```python
from build123d import *

# Parameters (mm, degrees)
F0_R     = 11.049
F1_DEPTH = 6.35


with BuildPart() as f1:
    # F0 (on Top) → F1 (new body)
    with BuildSketch(Plane.XY):
        with BuildLine():
            ThreePointArc((30.5423546194, 13.9698608404), (19.000422111, 19.0038325132), (13.9698381707, 30.547241977))
            ThreePointArc((13.9698381707, 30.547241977), (13.9699595426, 30.5136210859), (13.97, 30.48))
            ThreePointArc((13.97, 30.48), (9.8782817373, 20.6017182709), (1.15e-08, 16.51))
            ThreePointArc((1.15e-08, 16.51), (11.6743329615, 11.6743329533), (16.51, 0))
            ThreePointArc((16.51, 0), (20.623788609, 9.900302875), (30.5423546194, 13.9698608404))
        make_face()
        with BuildLine():
            ThreePointArc((1.15e-08, 16.51), (-9.8782817291, 20.6017182627), (-13.97, 30.48))
            ThreePointArc((-13.97, 30.48), (-18.9768088864, 19.0202694582), (-30.4173910664, 13.969859703))
            ThreePointArc((-30.4173910664, 13.969859703), (-20.5796074118, 9.8561212756), (-16.51, 0))
            ThreePointArc((-16.51, 0), (-11.6743329533, 11.6743329615), (1.15e-08, 16.51))
        make_face()
        with BuildLine():
            ThreePointArc((-30.4173910664, 13.969859703), (-40.3361211962, 9.9003926673), (-44.45, 2.241e-07))
            ThreePointArc((-44.45, 2.241e-07), (-40.2581741683, -9.9773849246), (-30.1982875449, -13.9671592707))
            ThreePointArc((-30.1982875449, -13.9671592707), (-20.5026149969, -9.7781740883), (-16.51, 0))
            ThreePointArc((-16.51, 0), (-20.5796074118, 9.8561212756), (-30.4173910664, 13.969859703))
        make_face()
        with Locations((-30.48, 0)):
            Circle(F0_R, mode=Mode.SUBTRACT)
        with BuildLine():
            ThreePointArc((-30.1982875449, -13.9671592707), (-18.895154623, -19.0895439026), (-13.97, -30.48))
            ThreePointArc((-13.97, -30.48), (-9.8782817214, -20.6017182551), (3.33e-08, -16.51))
            ThreePointArc((3.33e-08, -16.51), (-11.6743329456, -11.6743329692), (-16.51, 0))
            ThreePointArc((-16.51, 0), (-20.5026149969, -9.7781740883), (-30.1982875449, -13.9671592707))
        make_face()
        with BuildLine():
            ThreePointArc((13.9686715274, -30.6726545055), (18.8427220321, -19.1504715121), (30.2294023882, -13.9677521755))
            ThreePointArc((30.2294023882, -13.9677521755), (20.5135124382, -9.7892811626), (16.51, 0))
            ThreePointArc((16.51, 0), (11.6743329692, -11.6743329456), (3.33e-08, -16.51))
            ThreePointArc((3.33e-08, -16.51), (9.8782817449, -20.6017182786), (13.97, -30.48))
            ThreePointArc((13.97, -30.48), (13.9696678779, -30.5763295429), (13.9686715274, -30.6726545055))
        make_face()
        with BuildLine():
            ThreePointArc((3.33e-08, -16.51), (11.6743329692, -11.6743329456), (16.51, 0))
            Line((16.51, 0), (11.049, 0))
            ThreePointArc((11.049, 0), (7.8128228253, -7.8128228253), (0, -11.049))
            Line((0, -11.049), (0, -16.51))
        make_face()
        with BuildLine():
            Line((11.049, 0), (16.51, 0))
            ThreePointArc((16.51, 0), (11.6743329615, 11.6743329533), (1.15e-08, 16.51))
            Line((0, 16.51), (0, 11.049))
            ThreePointArc((0, 11.049), (7.8128228253, 7.8128228253), (11.049, 0))
        make_face()
        with BuildLine():
            Line((0, 11.049), (0, 16.51))
            ThreePointArc((1.15e-08, 16.51), (-11.6743329533, 11.6743329615), (-16.51, 0))
            Line((-16.51, 0), (-11.049, 0))
            ThreePointArc((-11.049, 0), (-7.8128228253, 7.8128228253), (0, 11.049))
        make_face()
        with BuildLine():
            ThreePointArc((-16.51, 0), (-11.6743329456, -11.6743329692), (3.33e-08, -16.51))
            Line((0, -16.51), (0, -11.049))
            ThreePointArc((0, -11.049), (-7.8128228253, -7.8128228253), (-11.049, 0))
            Line((-11.049, 0), (-16.51, 0))
        make_face()
        with BuildLine():
            ThreePointArc((-13.97, -30.48), (-9.8782816496, -40.3582818168), (2.364e-07, -44.45))
            ThreePointArc((2.364e-07, -44.45), (9.8099316986, -40.4261620774), (13.9686715274, -30.6726545055))
            ThreePointArc((13.9686715274, -30.6726545055), (13.9696678779, -30.5763295429), (13.97, -30.48))
            ThreePointArc((13.97, -30.48), (9.8782817449, -20.6017182786), (3.33e-08, -16.51))
            ThreePointArc((3.33e-08, -16.51), (-9.8782817214, -20.6017182551), (-13.97, -30.48))
        make_face()
        with BuildLine():
            ThreePointArc((11.049, -30.48), (-7.8128228253, -38.2928228253), (0, -19.431))
            ThreePointArc((0, -19.431), (7.8128228253, -22.6671771747), (11.049, -30.48))
        make_face(mode=Mode.SUBTRACT)
        with BuildLine():
            ThreePointArc((30.2294023882, -13.9677521755), (40.2692811626, -9.9664875618), (44.45, 0))
            ThreePointArc((44.45, 0), (40.5557673489, 9.6767666258), (31.0441571466, 13.9586040389))
            ThreePointArc((31.0441571466, 13.9586040389), (30.7932148695, 13.9624041517), (30.5423546194, 13.9698608404))
            ThreePointArc((30.5423546194, 13.9698608404), (20.623788609, 9.900302875), (16.51, 0))
            ThreePointArc((16.51, 0), (20.5135124382, -9.7892811626), (30.2294023882, -13.9677521755))
        make_face()
        with BuildLine():
            ThreePointArc((41.529, 0), (30.48, -11.049), (19.431, 0))
            ThreePointArc((19.431, 0), (30.48, 11.049), (41.529, 0))
        make_face(mode=Mode.SUBTRACT)
        with BuildLine():
            ThreePointArc((13.9698381707, 30.547241977), (9.8544794632, 40.382026788), (1.001e-07, 44.45))
            ThreePointArc((1.001e-07, 44.45), (-9.8782816978, 40.3582817686), (-13.97, 30.48))
            ThreePointArc((-13.97, 30.48), (-9.8782817291, 20.6017182627), (1.15e-08, 16.51))
            ThreePointArc((1.15e-08, 16.51), (9.8782817373, 20.6017182709), (13.97, 30.48))
            ThreePointArc((13.97, 30.48), (13.9699595426, 30.5136210859), (13.9698381707, 30.547241977))
        make_face()
        with BuildLine():
            ThreePointArc((11.049, 30.48), (7.8128228253, 22.6671771747), (0, 19.431))
            ThreePointArc((0, 19.431), (-7.8128228253, 38.2928228253), (11.049, 30.48))
        make_face(mode=Mode.SUBTRACT)
    extrude(amount=F1_DEPTH)


solid = f1.part
```
For this review, take the finished solid that the model builds, in its own axes (mm). Coordinates: 2 decimals unless noted, no trailing zeros. Loops run counter-clockwise (first coordinate to the right, second up) from the corner with the lowest first, then second, coordinate; pieces in that order, holes last. Notation, with made-up numbers: (6, 33.25) -> (24, 33.25) arc R21 ccw to (24, 72.25) -> close; hole circle Ø5 at (-36.75, 56). An arc over 180 degrees is marked (long way). Return JSON: item names as keys, results as strings. Group by question number.
(1) Consider section B-B, the plane z = 1.5. Give the boundary of the cut face in (x, y), plus the area to 3 significant figures.
(2) Consider section D-D, the plane x = 22. Give the boundary of the cut face in (y, z), plus the area to 3 significant figures.
(3) Consider section C-C, the plane y = -24. Give the boundary of the cut face in (x, z), plus the area to 3 significant figures.
(4) Mouldability with a two-part tool opening along X and no side actions: class faces 1 (the cylindrical face through (-41.52, 0.49, 3.13)), 2 (the flat face through (-7, 10, 6.35)), 3 (the cylindrical face through (18.7, -19.3, 3.1)) as pulls with the +X half, pulls with the -X half, needs draft (parallel to the pull), parting line crosses it, or undercut.
(5) Consider section A-A, the plane y = -7. Give the boundary of the cut face in (x, z).
(6) To check wall thickness, follow L1, parallel to Y at x = 30.48, z = 1.75; L2, parallel to X at y = -30.48, z = 2.5; L3, parallel to X at y = -7, z = 6. State the ranges of each line that lie inside material, in increasing order.
(7) For pin 1 Ø20 at (x, y) = (0, 30.48) entering from +Z; pin 2 Ø3 at (x, y) = (-21.5, 16) entering from -Z; pin 3 Ø2 at (x, z) = (-4.5, 5.5) entering from -Y; pin 4 Ø1 at (x, z) = (-12.5, 2) entering from -Y, all flat-tipped, find the tip position at first contact; note any pin that passes through.
Results below:
{
 "1": {"outline": "(-30.42, 13.97) arc R13.97 ccw (long way) to (-30.2, -13.97) arc R17.22 cw to (-13.97, -30.48) arc R13.97 ccw to (13.97, -30.67) arc R17.22 cw to (30.23, -13.97) arc R13.97 ccw to (31.04, 13.96) arc R17.22 cw to (13.97, 30.55) arc R13.97 ccw to (-13.97, 30.48) arc R17.22 cw to start; hole circle Ø22.1 at (-30.48, 0); hole circle Ø22.1 at (0, -30.48); hole circle Ø22.1 at (0, 0); hole circle Ø22.1 at (0, 30.48); hole circle Ø22.1 at (30.48, 0)", "area": "2,190 mm2"},
 "2": {"outline": "(-16.59, 0) -> (-7.08, 0) -> (-7.08, 6.35) -> (-16.59, 6.35) -> close; (7.08, 0) -> (16.61, 0) -> (16.61, 6.35) -> (7.08, 6.35) -> close", "area": "121 mm2"},
 "3": {"outline": "(-15.52, 0) -> (-8.95, 0) -> (-8.95, 6.35) -> (-15.52, 6.35) -> close; (8.95, 0) -> (15.52, 0) -> (15.52, 6.35) -> (8.95, 6.35) -> close", "area": "83.4 mm2"},
 "4": {"face 1": "undercut", "face 2": "needs draft", "face 3": "pulls with the +X half"},
 "5": {"outline": "(-42.57, 0) -> (-39.03, 0) -> (-39.03, 6.35) -> (-42.57, 6.35) -> close; (-21.93, 0) -> (-8.55, 0) -> (-8.55, 6.35) -> (-21.93, 6.35) -> close; (8.55, 0) -> (21.93, 0) -> (21.93, 6.35) -> (8.55, 6.35) -> close; (39.03, 0) -> (42.57, 0) -> (42.57, 6.35) -> (39.03, 6.35) -> close"},
 "6": {"L1": "y = -13.97 to -11.05, 11.05 to 13.97", "L2": "x = -13.97 to -11.05, 11.05 to 13.98", "L3": "x = -42.57 to -39.03, -21.93 to -8.55, 8.55 to 21.93, 39.03 to 42.57"},
 "7": {"pin 1": "passes through", "pin 2": "stops at z = 0", "pin 3": "stops at y = -44", "pin 4": "stops at y = -37.63"}
}
